The listing builds one solid part. Answer for the finished solid, in the listing's coordinates (mm). A direction names the side the tool comes from. Give positions to 0.01 mm unless a question says otherwise; leave off trailing zeros. Write each loop counter-clockwise with the first axis right and the second up, starting at its lowest first coordinate (ties: lowest second). Pieces come first, ordered by that corner, then holes. Notation, with made-up numbers: (40, 55) - (79, 55) arc R21 ccw to (79, 79) - close; hole circle Ø4 at (63.25, -27.75). An arc over 180 degrees is marked (long way). One line per question, with ' | ' between items. Start each with the question number.
1. A cutting plane is placed at D-D (z = 6.5). Determine the outline of the cut face in (x, y) (3 decimals).
2. A cutting plane is placed at B-B (y = -127). Determine the outline of the cut face in (x, z) (3 decimals).
3. Find the intervals of material crossed by L1, parallel to Z at x = 1, y = -127; L2, parallel to Z at x = 2.5, y = 12.7 (3 decimals); L3, parallel to X at y = 12, z = 45.5 (3 decimals), in increasing order. Write a range as from..to.
4. A cutting plane is placed at A-A (y = -101.6). Determine the outline of the cut face in (x, z) (3 decimals), then the cut area to 3 significant figures.
5. For faces 1 (the face through (50.8, -95, 2)), 2 (the face through (28.575, -25, 2)), 3 (the face through (27, -69, 3.175)), determine the directions among +Z, -Z, +X, -X, +Y, -Y from which every point of the face is accessible in a straight line to the end or side of a thin tool.
6. Given P1, Ø4, axis at y = -113, z = 13.5, coming from the -X side; P2, Ø7.5, axis at y = 12.7, z = 38.1, coming from the +X side (3 decimals); P3, Ø5, axis at y = 38.1, z = 12.7, coming from the +X side; P4, Ø1.6, axis at x = 16.5, z = 1.5, coming from the +Y side, each flat-ended and moving along its own axis, determine where each tip first touches the part or whether it passes through.
7. A cutting plane is placed at C-C (x = 15.5). Determine the outline of the cut face in (y, z) (3 decimals), then the cut area to 3 significant figures.
8. The mould has two halves that part along Z. Classify faces 4 (the face through (16, 0, 2)), 5 (the face through (1.61, 34.95, 12.29)), 6 (the face through (2, -46, 50.8)): +Z half, -Z half, draft (parallel to the pull), parting line (faces both ways), or undercut.
Autodesk Inventor part; units mm, degrees
ref_plane "YZ Plane" through (0, 0, 0) normal (1, 0, 0) x (0, 1, 0)
ref_plane "XZ Plane" through (0, 0, 0) normal (0, 1, 0) x (-1, 0, 0)
ref_plane "XY Plane" through (0, 0, 0) normal (0, 0, 1) x (1, 0, 0)
sketch "Sketch1" plane through (0, 0, 0) normal (0, 1, 0) x (-1, 0, 0)
  line L0 (0, 0) -> (-3.175, 0)
  line L1 (-3.175, 0) -> (-3.175, 50.8)
  line L2 (-3.175, 50.8) -> (0, 50.8)
  line L3 (0, 50.8) -> (0, 0)
  line L4 (0, 0) -> (-50.8, 0)
  line L5 (-50.8, 0) -> (-50.8, 3.175)
  line L6 (-50.8, 3.175) -> (0, 3.175)
  line L7 (0, 3.175) -> (0, 0)
  dimension "d0" = 3.175
  dimension "d1" = 50.8
  dimension "d2" = 50.8
  dimension "d3" = 3.175
extrude "Extrusion1" add sketch "Sketch1" against normal blind 139.7
sketch "Sketch3" plane through (0, 0, 0) normal (-1, 0, 0) x (0, 0, 1)
  line L0 (0, 0) -> (50.8, 0)
  line L1 (0, 0) -> (0, -139.7)
  line L2 (50.8, -139.7) -> (0, -139.7)
  line L3 (50.8, 0) -> (50.8, -139.7)
  point P0 (15.875, -127)
  point P1 (41.275, -127)
  dimension "d17" = 9.525
  dimension "d18" = 12.7
  dimension "d19" = 12.7
  dimension "d20" = 15.875
hole "Hole2" at (0, -127, 15.875) at (0, -127, 41.275) direction (1, 0, 0) diameter 6.35 end through all
sketch "Sketch4" plane through (50.8, 0, 0) normal (0, 0, -1) x (-1, 0, 0)
  line L0 (50.8, -139.7) -> (0, -139.7)
  line L1 (50.8, 0) -> (50.8, -139.7)
  line L2 (0, 0) -> (50.8, 0)
  line L3 (0, 0) -> (0, -139.7)
  point P0 (22.225, -63.5)
  point P1 (22.225, -101.6)
  dimension "d28" = 28.575
  dimension "d29" = 28.575
  dimension "d30" = 63.5
  dimension "d31" = 101.6
hole "Hole3" at (28.575, -63.5, 0) at (28.575, -101.6, 0) direction (0, 0, 1) diameter 6.35 end through all
sketch "Sketch5" plane through (0, 0, 0) normal (0, 1, 0) x (1, 0, 0)
  line L0 (0, 0) -> (0, -50.8)
  line L1 (0, -50.8) -> (3.175, -50.8)
  line L2 (3.175, -50.8) -> (3.175, -3.175)
  line L3 (3.175, -3.175) -> (50.8, -3.175)
  line L4 (50.8, -3.175) -> (50.8, 0)
  line L5 (50.8, 0) -> (0, 0)
  line L6 (0, 0) -> (3.175, 0)
  line L7 (3.175, 0) -> (3.175, -50.8)
  line L8 (3.175, -50.8) -> (0, -50.8)
  line L9 (0, -50.8) -> (0, 0)
extrude "Extrusion2" add sketch "Sketch5" along normal blind 50.8 contours L5 L7 L2 L1 L0
sketch "Sketch6" plane through (0, 0, 0) normal (0, 1, 0) x (1, 0, 0)
  line L0 (3.175, 0) -> (3.175, -3.175)
  line L1 (3.175, -3.175) -> (50.8, -3.175)
  line L2 (50.8, -3.175) -> (50.8, 0)
  line L3 (50.8, 0) -> (3.175, 0)
  line L4 (50.8, 0) -> (28.575, 0)
  line L5 (28.575, 0) -> (28.575, -3.175)
  line L6 (28.575, -3.175) -> (50.8, -3.175)
  line L7 (50.8, -3.175) -> (50.8, 0)
  point P0 (0, 0)
  dimension "d41" = 22.225
extrude "Extrusion3" cut sketch "Sketch6" against normal blind 50.8 contours L3 L2 L1 L5
sketch "Sketch7" plane through (0, -139.7, 0) normal (-1, 0, 0) x (0, 0, 1)
  circle A0 centre (15.875, 12.7) radius 3.175
  circle A1 centre (41.275, 12.7) radius 3.175
  line L0 (0, 190.5) -> (0, 0)
  line L1 (50.8, 0) -> (0, 0)
  line L2 (50.8, 0) -> (50.8, 190.5)
  line L3 (0, 190.5) -> (50.8, 190.5)
  point P0 (0, 139.7)
  point P1 (12.7, 177.8)
  point P2 (38.1, 177.8)
  point P3 (38.1, 152.4)
  point P4 (12.7, 152.4)
  dimension "d44" = 12.7
  dimension "d45" = 38.1
  dimension "d46" = 38.1
  dimension "d47" = 12.7
  dimension "d48" = 12.7
  dimension "d49" = 12.7
  dimension "d50" = 12.7
  dimension "d51" = 12.7
hole "Hole4" at (0, 38.1, 12.7) at (0, 38.1, 38.1) at (0, 12.7, 38.1) at (0, 12.7, 12.7) direction (1, 0, 0) diameter 6.35 end through all
properties part number "2x2 angle vertical left"
Determined:
1) outline: (0, -139.7) - (3.175, -139.7) - (3.175, 50.8) - (0, 50.8) - close
2) outline: (0, 0) - (50.8, 0) - (50.8, 3.175) - (3.175, 3.175) - (3.175, 12.7) - (0, 12.7) - close; (0, 19.05) - (3.175, 19.05) - (3.175, 38.1) - (0, 38.1) - close; (0, 44.45) - (3.175, 44.45) - (3.175, 50.8) - (0, 50.8) - close
3) L1: 0..12.7, 19.05..38.1, 44.45..50.8 | L2: 0..9.525, 15.875..34.925, 41.275..50.8 | L3: 0..3.175
4) outline: (0, 0) - (25.4, 0) - (25.4, 3.175) - (3.175, 3.175) - (3.175, 50.8) - (0, 50.8) - close; (31.75, 0) - (50.8, 0) - (50.8, 3.175) - (31.75, 3.175) - close | area: 292 mm2
5) face 1: +Z, -Z, +X, +Y, -Y | face 2: +Z, -Z, +X, +Y | face 3: +Z, +X, +Y, -Y
6) P1: x = 0 | P2: x = 3.175 | P3: through | P4: y = 0
7) outline: (-139.7, 0) - (0, 0) - (0, 3.175) - (-139.7, 3.175) - close | area: 444 mm2
8) face 4: draft | face 5: undercut | face 6: +Z half
